```python
from build123d import *

# Parameters (mm, degrees)
CYLINDER093_R     = 1.5
CYLINDER093_DEPTH = 14
CYLINDER090_R     = 11.7
CYLINDER090_DEPTH = 33
CYLINDER094_R     = 1.5
CYLINDER094_DEPTH = 14
CYLINDER088_R     = 14
CYLINDER088_DEPTH = 33
BOX016_W          = 47
BOX016_H          = 10
BOX016_DEPTH      = 5
CYLINDER084_R     = 17
CYLINDER084_DEPTH = 5


with BuildPart() as obj1:
    # Cylinder093 → Cylinder093 (new body)
    with BuildSketch(Plane(origin=(53.66, 148, -15), x_dir=(1, 0, 0), z_dir=(0, 0, 1))):
        Circle(CYLINDER093_R)
    extrude(amount=CYLINDER093_DEPTH)


with BuildPart() as obj2:
    # Cylinder090 → Cylinder090 (new body)
    with BuildSketch(Plane(origin=(73.66, 148, -10), x_dir=(1, 0, 0), z_dir=(0, 0, 1))):
        Circle(CYLINDER090_R)
    extrude(amount=CYLINDER090_DEPTH)


with BuildPart() as fusion039:
    # Cylinder094 → Cylinder094 (new body)
    with BuildSketch(Plane(origin=(93.66, 148, -14), x_dir=(1, 0, 0), z_dir=(0, 0, 1))):
        Circle(CYLINDER094_R)
    extrude(amount=CYLINDER094_DEPTH)

    # Fusion039: union obj1, obj2
    add(obj1.part)
    add(obj2.part)


with BuildPart() as obj3:
    # Cylinder088 → Cylinder088 (new body)
    with BuildSketch(Plane(origin=(73.66, 148, -10), x_dir=(1, 0, 0), z_dir=(0, 0, 1))):
        Circle(CYLINDER088_R)
    extrude(amount=CYLINDER088_DEPTH)


with BuildPart() as obj4:
    # Box016 → Box016 (new body)
    with BuildSketch(Plane(origin=(50, 143, 7), x_dir=(1, 0, 0), z_dir=(0, 0, 1))):
        with Locations((23.5, 5)):
            Rectangle(BOX016_W, BOX016_H)
    extrude(amount=BOX016_DEPTH)


with BuildPart() as obj5:
    # Cylinder084 → Cylinder084 (new body)
    with BuildSketch(Plane(origin=(73.66, 148, -10), x_dir=(1, 0, 0), z_dir=(0, 0, 1))):
        Circle(CYLINDER084_R)
    extrude(amount=CYLINDER084_DEPTH)

    # Fusion038: union obj3, obj4
    add(obj3.part)
    add(obj4.part)

    # Cut010: cut Fusion039
    add(fusion039.part, mode=Mode.SUBTRACT)


with BuildPart() as obj5_1:
    # Cut010 placement: moved
    add(obj5.part.moved(Location((0, 0, 5))))


solid = obj5_1.part
```
Part model, mm, in its own coordinate system. A direction names the side the tool comes from. Round coordinates to 2 decimals unless told otherwise and drop trailing zeros. Write each loop counter-clockwise with the first axis right and the second up, starting at its lowest first coordinate (ties: lowest second). Pieces come first, ordered by that corner, then holes. Notation, with made-up numbers: M 80,-7 L 109,-7 A23 cw 109,26 Z; hole C -33,22 d11. An arc over 180 degrees is marked long. One line per question, with ' | ' between items.
(1) Saw through at C-C on x = 75. Write the cut outline in (y, z), then the cut area to 3 significant figures.
Answer key:
outline: M 131.05,-5 L 136.38,-5 L 136.38,28 L 134.06,28 L 134.06,0 L 131.05,0 Z; M 159.62,-5 L 164.95,-5 L 164.95,0 L 161.94,0 L 161.94,28 L 159.62,28 Z | area: 183 mm^2
(2) Saw through at A-A on y = 148. Write the cut outline in (x, z), then the cut area to 3 significant figures.
Answer key:
outline: M 50,12 L 59.66,12 L 59.66,0 L 56.66,0 L 56.66,-5 L 61.96,-5 L 61.96,28 L 59.66,28 L 59.66,17 L 50,17 Z; M 85.36,-5 L 90.66,-5 L 90.66,0 L 87.66,0 L 87.66,12 L 97,12 L 97,17 L 87.66,17 L 87.66,28 L 85.36,28 Z | area: 277 mm^2
(3) 3-axis set-ups, long thin cutter, end or side, ignore diameter. For faces 1 (the face through (55, 143, 14)), 2 (the face through (65.04, 155.91, 11.27)), 3 (the face through (55, 153, 14)), 4 (the face through (76, 162, 0)), 5 (the face through (92, 153, 14)): which of +Z, -Z, +X, -X, +Y, -Y reach the whole face in a straight line?
Answer key:
face 1: +Z, -X, -Y | face 2: +Z, -Z | face 3: +Z, -X, +Y | face 4: none | face 5: +Z, +X, +Y
(4) Pin check, flat tips, straight feed: pin 1 (1.5 mm diameter, centred on x = 52.5, z = 15.5, fed in from +Y); pin 2 (11 mm diameter, centred on x = 56, y = 148.5, fed in from -Z); pin 3 (1.5 mm diameter, centred on x = 55, z = 15, fed in from -Y); pin 4 (8 mm diameter, centred on x = 53, y = 148.5, fed in from +Z). Stop position of each tip, or through.
Answer key:
pin 1: stops at y = 153 | pin 2: stops at z = -5 | pin 3: stops at y = 143 | pin 4: stops at z = 17
(5) Saw through at B-B on z = 14. Write the cut outline in (x, y), then the cut area to 3 significant figures.
Answer key:
outline: M 50,143 L 60.58,143 A14 ccw 86.74,143 L 97,143 L 97,153 L 86.74,153 A14 ccw 60.58,153 L 50,153 Z; hole C 73.66,148 d23.4 | area: 382 mm^2
(6) Two-plate mould, pull along Z, no slides. Class faces 6 (the face through (92, 143, 14)), 7 (the face through (92, 148, 12)), 8 (the face through (66.3, 138.7, 28)): released by +Z, released by -Z, zero draft, split by the parting line, or undercut.
Answer key:
face 6: zero draft | face 7: undercut | face 8: released by +Z
(7) Probe line 1 along Y through (x, z) = (73.66, 15.5); line 2 along X through (y, z) = (139, 5); line 3 along Z through (x, y) = (93, 149.5). List the from-to ranges inside material, lowest first.
Answer key:
line 1: y = 134 to 136.3, 159.7 to 162 | line 2: x = 62.94 to 66.18, 81.14 to 84.38 | line 3: z = 12 to 17
(8) Saw through at D-D on y = 139.5. Write the cut outline in (x, z).
Answer key:
outline: M 58.94,-5 L 65.62,-5 L 65.62,28 L 62.54,28 L 62.54,0 L 58.94,0 Z; M 81.7,-5 L 88.38,-5 L 88.38,0 L 84.78,0 L 84.78,28 L 81.7,28 Z
